Autodesk Inventor part; units mm, degrees
ref_plane "YZ Plane" through (0, 0, 0) normal (1, 0, 0) x (0, 1, 0)
ref_plane "XZ Plane" through (0, 0, 0) normal (0, 1, 0) x (-1, 0, 0)
ref_plane "XY Plane" through (0, 0, 0) normal (0, 0, 1) x (1, 0, 0)
sketch "Sketch1" plane through (0, 0, 0) normal (0, 1, 0) x (-1, 0, 0)
  circle A0 centre (0, 0) radius 34.925
  dimension "d0" = 69.85
extrude "Extrusion1" add sketch "Sketch1" along normal blind 2.54
sketch "Sketch2" plane through (0, 0, 0) normal (0, -1, 0) x (1, 0, 0)
  line L0 (0, 0) -> (15.24, 0)
  line L1 (15.24, 0) -> (15.24, -27.94)
  line L2 (15.24, -27.94) -> (12.7, -27.94)
  line L3 (12.7, -27.94) -> (12.7, 27.94)
  line L4 (12.7, 27.94) -> (15.24, 27.94)
  line L5 (15.24, 27.94) -> (15.24, -27.94)
  line L6 (0, 0) -> (0, -3.81)
  line L7 (0, -3.81) -> (-3.81, -3.81)
  arc A0 (-3.81, -6.985) -> (-6.985, -3.81) centre (-6.985, -6.985) ccw
  arc A1 (-29.21, -3.81) -> (-3.81, -29.21) centre (-3.81, -3.81) ccw
  line L8 (-3.81, -3.81) -> (-3.81, -29.21) construction
  line L9 (-3.81, -3.81) -> (-29.21, -3.81) construction
  line L10 (-3.81, -29.21) -> (-3.81, -6.985)
  line L11 (-29.21, -3.81) -> (-6.985, -3.81)
  circle A2 centre (0, 0) radius 34.925
  line L12 (-34.925, 0) -> (0, 0)
  arc A3 (-6.985, 3.81) -> (-3.81, 6.985) centre (-6.985, 6.985) ccw
  arc A4 (-3.81, 29.21) -> (-29.21, 3.81) centre (-3.81, 3.81) ccw
  line L13 (-3.81, 3.81) -> (-3.81, 29.21) construction
  line L14 (-3.81, 3.81) -> (-29.21, 3.81) construction
  line L15 (-6.985, 3.81) -> (-29.21, 3.81)
  line L16 (-3.81, 6.985) -> (-3.81, 29.21)
  line L17 (15.24, 0) -> (22.86, 0)
  line L18 (22.86, 0) -> (22.86, -22.0337)
  line L19 (22.86, 22.0337) -> (22.86, 0)
  arc A5 (15.0804, -27.94) -> (15.24, -27.8533) centre (0, 0) ccw
  arc A6 (22.86, -22.0337) -> (22.86, 22.0337) centre (0, 0) ccw
  arc A7 (15.24, 27.8533) -> (15.0804, 27.94) centre (0, 0) ccw
  circle A8 centre (0, 0) radius 4.445
  dimension "d3" = 15.24
  dimension "d4" = 27.94
  dimension "d5" = 2.54
  dimension "d6" = 55.88
  dimension "d7" = 3.81
  dimension "d8" = 3.81
  dimension "d9" = 25.4
  dimension "d11" = 3.175
  dimension "d13" = 25.4
  dimension "d14" = 90
  dimension "d19" = 7.62
  dimension "d20" = 8.89
extrude "Extrusion2" cut sketch "Sketch2" against normal blind 2.54 contours L12 A8 L0 | L0 A8 L7 L6 | L6 L7 A8 L12 | L19 A6 L18 | L3 L4 A7 L5 L0 | L0 L1 A5 L2 L3 | L1 L2 A5 | A7 L4 L5 | L10 A1 L11 A0 | L15 A4 L16 A3
properties part number "fixpart"
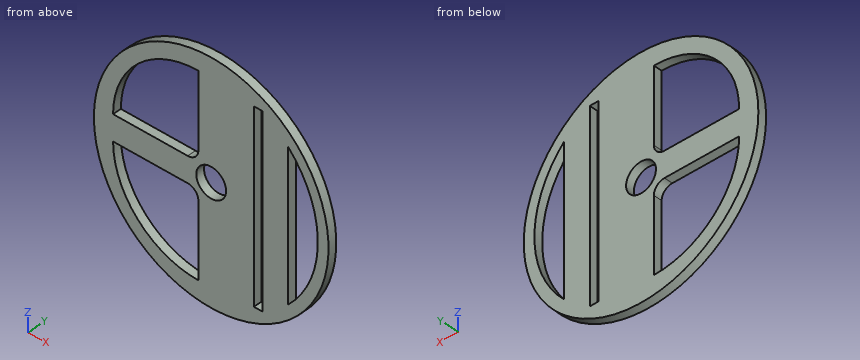
The listing builds one solid part. Answer for the finished solid, in the listing's coordinates (mm). Coordinates: 2 decimals unless noted, no trailing zeros. Order: outer loops, then holes, each group sorted by start corner. A loop starts at its lowest first (then second) coordinate and runs counter-clockwise, first axis right, second up.
Q1. A cutting plane is placed at D-D, the plane x = -25.5. Write down the section's boundary in (y, z), and give its area (3 significant figures).
Q2. Given P1, Ø0.8, axis at x = -20.5, y = 1.5, coming from the +Z side; P2, Ø0.8, axis at y = 1, z = -21.5, coming from the -X side; P3, Ø1.3, axis at x = -16, y = 1.5, coming from the -Z side, each flat-ended and moving along its own axis, determine where each tip first touches the part or whether it passes through.
Q3. A cutting plane is placed at B-B, the plane z = 0. Write down the section's boundary in (x, y) (3 decimals), and give its area (3 significant figures).
Q4. A cutting plane is placed at C-C, the plane y = 2.1. Write down the section's boundary in (x, z) (3 decimals), and give its area (3 significant figures).
Q5. Consider line 1 (X direction, y = 2.4, z = -15); line 2 (Z direction, x = 0, y = 1.65) (3 decimals); line 3 (X direction, y = 1.8, z = 5.5). Determine where each line is inside the solid, lowest interval first.
Q6. A cutting plane is placed at A-A, the plane x = 0. Write down the section's boundary in (y, z) (3 decimals), and give its area (3 significant figures).
Answers follow:
1. outline: (0, -23.86) - (2.54, -23.86) - (2.54, -17.03) - (0, -17.03) - close; (0, -3.81) - (2.54, -3.81) - (2.54, 3.81) - (0, 3.81) - close; (0, 17.03) - (2.54, 17.03) - (2.54, 23.86) - (0, 23.86) - close
1. area: 54.1 mm2
2. P1: stops at z = 28.56
2. P2: stops at x = -27.83
2. P3: stops at z = -31.37
3. outline: (-34.925, 0) - (-4.445, 0) - (-4.445, 2.54) - (-34.925, 2.54) - close; (4.445, 0) - (12.7, 0) - (12.7, 2.54) - (4.445, 2.54) - close; (15.24, 0) - (22.86, 0) - (22.86, 2.54) - (15.24, 2.54) - close; (31.75, 0) - (34.925, 0) - (34.925, 2.54) - (31.75, 2.54) - close
3. area: 126 mm2
4. outline: circle Ø69.85 at (0, 0); hole (-29.21, -3.81) arc R25.4 ccw to (-3.81, -29.21) - (-3.81, -6.985) arc R3.175 ccw to (-6.985, -3.81) - close; hole (-29.21, 3.81) - (-6.985, 3.81) arc R3.175 ccw to (-3.81, 6.985) - (-3.81, 29.21) arc R25.4 ccw to start; hole circle Ø8.89 at (0, 0); hole (12.7, -27.94) - (15.24, -27.94) - (15.24, 27.94) - (12.7, 27.94) - close; hole (22.86, -22.034) arc R31.75 ccw to (22.86, 22.034) - close
4. area: 2,350 mm2
5. line 1: x = -31.54 to -26.61, -3.81 to 12.7, 15.24 to 22.86, 27.98 to 31.54
5. line 2: z = -34.925 to -4.445, 4.445 to 34.925
5. line 3: x = -34.49 to -29.15, -4.18 to 12.7, 15.24 to 22.86, 31.27 to 34.49
6. outline: (0, -34.925) - (2.54, -34.925) - (2.54, -4.445) - (0, -4.445) - close; (0, 4.445) - (2.54, 4.445) - (2.54, 34.925) - (0, 34.925) - close
6. area: 155 mm2
